```python
from build123d import *

# Parameters (mm, degrees)
F0_R      = 8.5
F1_DEPTH  = 20
F2_R      = 10
F3_DEPTH  = 8.83
F4_R      = 16
F5_DEPTH  = 35.4
F6_R      = 22.5
F7_DEPTH  = 59.13
F8_R      = 11.5
F9_DEPTH  = 35.4
F12_W     = 20
F12_H     = 4
F13_DEPTH = 4
F15_W     = 20
F15_H     = 4
F16_DEPTH = 4


with BuildPart() as f1:
    # F0 (on Front) → F1 (new body)
    with BuildSketch(Plane.XZ):
        Circle(F0_R)
    extrude(amount=F1_DEPTH)

    # F2 (on face) → F3 (join)
    with BuildSketch(Plane.XZ.offset(20)):
        Circle(F2_R)
    extrude(amount=F3_DEPTH)

    # F4 (on face) → F5 (join)
    with BuildSketch(Plane.XZ.offset(28.83)):
        Circle(F4_R)
    extrude(amount=F5_DEPTH)

    # F6 (on face) → F7 (join)
    with BuildSketch(Plane.XZ.offset(64.23)):
        Circle(F6_R)
    extrude(amount=F7_DEPTH)

    # F8 (on face) → F9 (join)
    with BuildSketch(Plane.XZ.offset(123.36)):
        Circle(F8_R)
    extrude(amount=F9_DEPTH)

    # F12 (on offset) → F13 (cut)
    with BuildSketch(Plane.YZ.offset(11.5)):
        with Locations((-141.06, 2)):
            Rectangle(F12_W, F12_H)
        with Locations((-141.06, -2)):
            Rectangle(F12_W, F12_H)
    extrude(amount=-F13_DEPTH, mode=Mode.SUBTRACT)

    # F15 (on offset) → F16 (cut)
    with BuildSketch(Plane.YZ.offset(16)):
        with Locations((-46.53, -2)):
            Rectangle(F15_W, F15_H)
        with Locations((-46.53, 2)):
            Rectangle(F15_W, F15_H)
    extrude(amount=-F16_DEPTH, mode=Mode.SUBTRACT)


solid = f1.part
```
Part model, mm, in its own coordinate system. A direction names the side the tool comes from. Coordinates: 2 decimals unless noted, no trailing zeros. Loops run counter-clockwise (first coordinate to the right, second up) from the corner with the lowest first, then second, coordinate; pieces in that order, holes last. Notation, with made-up numbers: (89.5, 80) - (96.5, 80) arc R23 ccw to (96.5, 91) - close; hole circle Ø5 at (39, 71). An arc over 180 degrees is marked (long way). Write item = value, one per line. Start each with the question number.
Item 1: 3-axis set-ups, long thin cutter, end or side, ignore diameter. For faces 1 (the cylindrical face through (-11.49, -140.81, 0.51)), 2 (the flat face through (10, -151.06, 0)), 3 (the cylindrical face through (10.382, -93.381, -19.961)), 4 (the flat face through (0, 0, 0)), 5 (the flat face through (-5.3, -64.23, 15.3)): which of +Z, -Z, +X, -X, +Y, -Y reach the whole face in a straight line?
Item 2: Cut at B-B, the plane x = 0. Give the cut face in (y, z).
Item 3: Flat gauge pins, fed straight in: pin 1 Ø1.6 at (x, y) = (8.5, -146) entering from +Z; pin 2 Ø4 at (x, z) = (-10.5, 3.5) entering from +Y; pin 3 Ø1.5 at (y, z) = (-120.5, 3) entering from -X. Where does each tip first touch, or does it go through?
Item 4: Cut at D-D, the plane z = 18. Give the cut face in (x, y).
Item 5: Wall check: L1, parallel to Y at x = 13, z = 1.5; L2, parallel to Y at x = -17, z = -4; L3, parallel to Y at x = -9.5, z = 4.5. Give the ranges that are in metal, low to high. Write a range as from..to.
Item 6: Mould opens along Z. For faces 6 (the flat face through (10, -123.36, -10)), 7 (the flat face through (14, -47, -4)), 8 (the cylindrical face through (-3.47, -46.28, -15.62)) say: released by +Z, released by -Z, zero draft, split by the parting line, or undercut.
Item 7: Cut at A-A, the plane z = 0. Give the cut face in (x, y).
Item 8: Cut at C-C, the plane y = -24. Give the cut face in (x, z).
The answers:
q1.face_1 = -Y
q1.face_2 = +X
q1.face_3 = +Y, -Y
q1.face_4 = +Z, -Z, +X, -X, +Y
q1.face_5 = +Y
q2.outline = (-158.76, -11.5) - (-123.36, -11.5) - (-123.36, -22.5) - (-64.23, -22.5) - (-64.23, -16) - (-28.83, -16) - (-28.83, -10) - (-20, -10) - (-20, -8.5) - (0, -8.5) - (0, 8.5) - (-20, 8.5) - (-20, 10) - (-28.83, 10) - (-28.83, 16) - (-64.23, 16) - (-64.23, 22.5) - (-123.36, 22.5) - (-123.36, 11.5) - (-158.76, 11.5) - close
q3.pin_1 = 8.54
q3.pin_2 = -20
q3.pin_3 = -22.39
q4.outline = (-13.5, -123.36) - (13.5, -123.36) - (13.5, -64.23) - (-13.5, -64.23) - close
q5.L1 = -123.36..-56.53, -36.53..-28.83
q5.L2 = -123.36..-64.23
q5.L3 = -158.76..-28.83
q6.face_6 = zero draft
q6.face_7 = undercut
q6.face_8 = split by the parting line
q7.outline = (-22.5, -123.36) - (-11.5, -123.36) - (-11.5, -158.76) - (11.5, -158.76) - (11.5, -151.06) - (7.5, -151.06) - (7.5, -131.06) - (11.5, -131.06) - (11.5, -123.36) - (22.5, -123.36) - (22.5, -64.23) - (16, -64.23) - (16, -56.53) - (12, -56.53) - (12, -36.53) - (16, -36.53) - (16, -28.83) - (10, -28.83) - (10, -20) - (8.5, -20) - (8.5, 0) - (-8.5, 0) - (-8.5, -20) - (-10, -20) - (-10, -28.83) - (-16, -28.83) - (-16, -64.23) - (-22.5, -64.23) - close
q8.outline = circle Ø20 at (0, 0)
